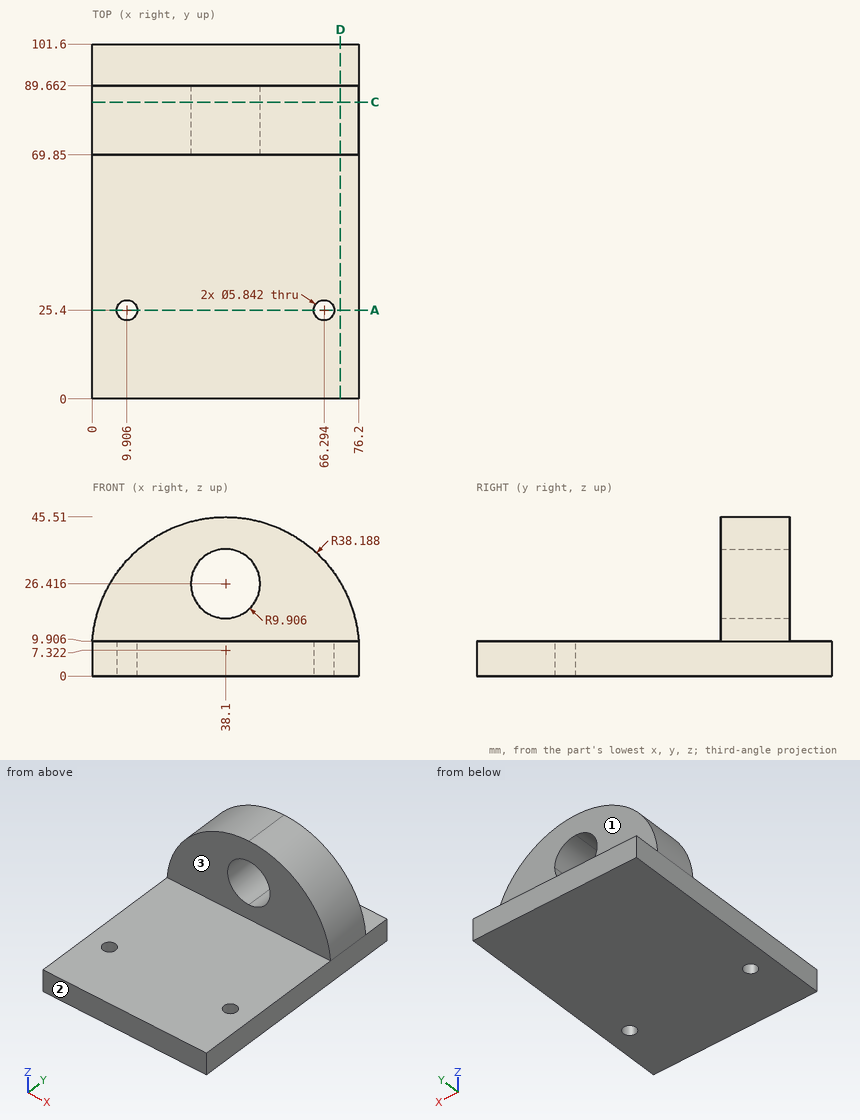
Check sheet for the drawn part. Datum: minimum x, y, z corner. Units: mm. A direction names the side the tool comes from. Coordinates: 2 decimals unless noted, no trailing zeros. Order: outer loops, then holes, each group sorted by start corner. A loop starts at its lowest first (then second) coordinate and runs counter-clockwise, first axis right, second up. Notation, with made-up numbers: (-35.75, 52.5) - (5.25, 52.5) arc R20 ccw to (5.25, 68.5) - close; hole circle Ø2 at (-34.75, 13.5). An arc over 180 degrees is marked (long way). Return JSON: item names as keys, results as strings.
(1) Section check A-A, the plane y = 25.4. Record the cut outline in (x, z) (1 decimal).
Filled sheet:
{"outline": "(0, 0) - (7, 0) - (7, 9.9) - (0, 9.9) - close; (12.8, 0) - (63.4, 0) - (63.4, 9.9) - (12.8, 9.9) - close; (69.2, 0) - (76.2, 0) - (76.2, 9.9) - (69.2, 9.9) - close"}
(2) Thickness scan on line 1 along X through (y, z) = (25, 5); line 2 along Y through (x, z) = (10.5, 33); line 3 along Z through (x, y) = (65.5, 62). Record the ranges inside material, lowest first.
Filled sheet:
{"line 1": "x = 0 to 7.01, 12.8 to 63.4, 69.19 to 76.2", "line 2": "y = 69.85 to 89.66", "line 3": "z = 0 to 9.91"}
(3) Section check C-C, the plane y = 85. Record the cut outline in (x, z) (1 decimal), and give its area (3 significant figures).
Filled sheet:
{"outline": "(0, 0) - (76.2, 0) - (76.2, 9.9) arc R38.2 ccw to (0, 9.9) - close; hole circle Ø19.8 at (38.1, 26.4)", "area": "2,540 mm^2"}
(4) Access from +Z, -Z, +X, -X, +Y, -Y to the whole of each face (thin tool, end or side, straight path). Record for the marked faces 1, 2 and 3.
Filled sheet:
{"face 1": "+Z, +X, -X, +Y", "face 2": "+Z, -Z, +X, -X, -Y", "face 3": "+Z, +X, -X, -Y"}
(5) Section check D-D, the plane x = 71. Record the cut outline in (y, z), and give its area (3 significant figures).
Filled sheet:
{"outline": "(0, 0) - (101.6, 0) - (101.6, 9.91) - (89.66, 9.91) - (89.66, 26.71) - (69.85, 26.71) - (69.85, 9.91) - (0, 9.91) - close", "area": "1,340 mm^2"}
(6) Go/stop test with flat-tipped pins: pin 1 (1 mm diameter, centred on x = 56.5, z = 40.5, fed in from -Y); pin 2 (6 mm diameter, centred on x = 38, z = 12, fed in from -Y); pin 3 (1.5 mm diameter, centred on x = 24.5, z = 39.5, fed in from +Y); pin 4 (3.5 mm diameter, centred on x = 39, y = 98, fed in from +Z). Record where each tip stops, or that it passes through.
Filled sheet:
{"pin 1": "stops at y = 69.85", "pin 2": "stops at y = 0", "pin 3": "stops at y = 89.66", "pin 4": "stops at z = 9.91"}
